Autodesk Inventor part; units mm, degrees
ref_plane "YZ Plane" through (0, 0, 0) normal (1, 0, 0) x (0, 1, 0)
ref_plane "XZ Plane" through (0, 0, 0) normal (0, 1, 0) x (-1, 0, 0)
ref_plane "XY Plane" through (0, 0, 0) normal (0, 0, 1) x (1, 0, 0)
sketch "スケッチ1" plane through (0, 0, 0) normal (0, 0, 1) x (1, 0, 0)
  line L0 (-19.75, 10) -> (19.75, 10) construction
  line L1 (19.75, 10) -> (19.75, -10) construction
  line L2 (19.75, -10) -> (-19.75, -10) construction
  line L3 (-19.75, -10) -> (-19.75, 10) construction
  line L4 (-19.75, 10) -> (19.75, -10) construction
  line L5 (19.75, 10) -> (-19.75, -10) construction
  line L6 (-19.75, 5) -> (-21.75, 5)
  line L7 (-21.75, 5) -> (-21.75, -5)
  line L8 (-19.75, 0) -> (19.75, 0) construction
  line L9 (0, 10) -> (0, -10) construction
  circle A0 centre (0, 0) radius 2.75
  arc A1 (-19.75, 5) -> (-19.75, 7.1) centre (-19.75, 6.05) ccw
  line L10 (-16.75, 10) -> (-11.75, 3)
  line L11 (-19.75, -5) -> (-21.75, -5)
  arc A2 (-19.75, -7.1) -> (-19.75, -5) centre (-19.75, -6.05) ccw
  line L12 (-16.75, -10) -> (-11.75, -3)
  line L13 (-19.75, 7.1) -> (-19.75, 10)
  line L14 (-16.75, 10) -> (-19.75, 10)
  line L15 (-16.75, -10) -> (-19.75, -10)
  line L16 (-19.75, -7.1) -> (-19.75, -10)
  line L17 (19.75, 5) -> (21.75, 5)
  line L18 (21.75, 5) -> (21.75, -5)
  arc A3 (19.75, 7.1) -> (19.75, 5) centre (19.75, 6.05) ccw
  line L19 (16.75, 10) -> (11.75, 3)
  line L20 (19.75, -5) -> (21.75, -5)
  arc A4 (19.75, -5) -> (19.75, -7.1) centre (19.75, -6.05) ccw
  line L21 (16.75, -10) -> (11.75, -3)
  line L22 (19.75, 7.1) -> (19.75, 10)
  line L23 (16.75, 10) -> (19.75, 10)
  line L24 (16.75, -10) -> (19.75, -10)
  line L25 (19.75, -7.1) -> (19.75, -10)
  arc A5 (5.1962, 3) -> (-5.1962, 3) centre (0, 0) ccw
  arc A6 (-5.1962, -3) -> (5.1962, -3) centre (0, 0) ccw
  line L26 (-2.0265, -3.51) -> (-2.5515, -2.6007) construction
  line L27 (-4.053, 0) -> (-3.528, 0.9093) construction
  line L28 (-2.0265, 3.51) -> (-0.9765, 3.51) construction
  line L29 (2.0265, 3.51) -> (2.5515, 2.6007) construction
  line L30 (4.053, 0) -> (3.528, -0.9093) construction
  line L31 (2.0265, -3.51) -> (0.9765, -3.51) construction
  arc A7 (-3.528, 0.9093) -> (-3.528, -0.9093) centre (-3.003, 0) ccw
  arc A8 (-2.5515, -2.6007) -> (-0.9765, -3.51) centre (-1.5015, -2.6007) ccw
  arc A9 (0.9765, -3.51) -> (2.5515, -2.6007) centre (1.5015, -2.6007) ccw
  arc A10 (3.528, -0.9093) -> (3.528, 0.9093) centre (3.003, 0) ccw
  arc A11 (2.5515, 2.6007) -> (0.9765, 3.51) centre (1.5015, 2.6007) ccw
  arc A12 (-0.9765, 3.51) -> (-2.5515, 2.6007) centre (-1.5015, 2.6007) ccw
  line L32 (-2.5515, 2.6007) -> (-2.0265, 3.51) construction
  line L33 (-3.528, 0.9093) -> (-2.5515, 2.6007)
  line L34 (-3.528, -0.9093) -> (-4.053, 0) construction
  line L35 (-2.5515, -2.6007) -> (-3.528, -0.9093)
  line L36 (-0.9765, -3.51) -> (-2.0265, -3.51) construction
  line L37 (0.9765, -3.51) -> (-0.9765, -3.51)
  line L38 (2.5515, -2.6007) -> (2.0265, -3.51) construction
  line L39 (3.528, -0.9093) -> (2.5515, -2.6007)
  line L40 (3.528, 0.9093) -> (4.053, 0) construction
  line L41 (2.5515, 2.6007) -> (3.528, 0.9093)
  line L42 (0.9765, 3.51) -> (2.0265, 3.51) construction
  line L43 (-0.9765, 3.51) -> (0.9765, 3.51)
  line L44 (-11.75, 3) -> (-5.1962, 3)
  line L45 (-5.1962, -3) -> (-11.75, -3)
  line L46 (5.1962, -3) -> (11.75, -3)
  line L47 (11.75, 3) -> (5.1962, 3)
  point P0 (0, 0)
  dimension "d0" = 39.5
  dimension "d3" = 5.5
  dimension "d4" = 2
  dimension "d5" = 10
  dimension "d6" = 1.05
  dimension "d7" = 3
  dimension "d9" = 5
  dimension "d11" = 8
  dimension "d12" = 6
  dimension "d14" = 1.05
  dimension "d17" = 360
  dimension "d19" = 7.02
  dimension "d20" = 6
extrude "押し出し1" add sketch "スケッチ1" along normal blind 3 contours A1 L13 L14 L10 L44 A5 L47 L19 L23 L22 A3 L17 L18 L20 A4 L25 L24 L21 L46 A6 L45 L12 L15 L16 A2 L11 L7 L6
extrude "押し出し2" add sketch "スケッチ1" along normal blind 0.6 contours L33 A12 L43 A11 L41 A10 L39 A9 L37 A8 L35 A7
fillet "フィレット1" radius 2 12 edges at (-11.75, 3, 1.5) (-11.75, -3, 1.5) (-16.75, 10, 1.5) (-16.75, -10, 1.5) (-5.1962, -3, 1.5) (-5.1962, 3, 1.5) (5.1962, 3, 1.5) (5.1962, -3, 1.5) (11.75, 3, 1.5) (11.75, -3, 1.5) (16.75, 10, 1.5) (16.75, -10, 1.5)
properties part number "Ankle_front_frame" material "アルミニウム 2014-T4"
Source: CAD feature listing. Evaluate the final solid. Frame: model axes, mm. A direction names the side the tool comes from. Give positions to 0.01 mm unless a question says otherwise; leave off trailing zeros. Loops run counter-clockwise (first coordinate to the right, second up) from the corner with the lowest first, then second, coordinate; pieces in that order, holes last. Notation, with made-up numbers: (1, 36) -> (16, 36) arc R29 cw to (16, 66) -> close; hole circle Ø6 at (67, -13). An arc over 180 degrees is marked (long way). Use a Markdown table: item, result. Add a question column.
1) Section query B-B, the plane y = -7.5. Return the cut outline in (x, z), then the cut area to 3 significant figures.
2) Reachability of faces 4 (the face through (21, 5, 1)), 5 (the face through (-5.37, -3.2, 1.52)), 6 (the face through (0, 3.51, 2)), 7 (the face through (-21, -5, 1)), 8 (the face through (16.876, 9.784, 1.521)) from +Z, -Z, +X, -X, +Y, -Y: full face, straight path, thin tool, end or side. Return the list, or none.
3) Section query D-D, the plane y = 1.5. Return the cut outline in (x, z).
4) Section query C-C, the plane x = 10. Return the cut outline in (y, z), then the cut area to 3 significant figures.
5) Section query A-A, the plane x = 0. Return the cut outline in (y, z).
6) Line query: line 1 along Y through (x, z) = (19, 2.75); line 2 along X through (y, z) = (-3.75, 2.2); line 3 along X through (y, z) = (-5.5, 2.7). Output: solid intervals per line, ascending. Write a range as [from, to].
7) Pull-direction query (X, two-part tool) for faces 1 (the face through (14.28, 6.54, 1.48)), 2 (the face through (21.75, 0, 1)), 3 (the face through (-5, 0, 3)); classes: +X half, -X half, draft (parallel to the pull), parting line (faces both ways), or undercut.
8) First-contact query: pin 1 (0.9 mm diameter, centred on x = 7.5, z = 1.5, fed in from -Y); pin 2 (7 mm diameter, centred on x = 0, y = 0, fed in from -Z); pin 3 (1.5 mm diameter, centred on y = 8, z = 2, fed in from -X); pin 4 (1 mm diameter, centred on x = 20.5, z = 1, fed in from +Y). Flat tips, straight axial feed; report the tip coordinate or a pass-through.
Numbers:
| question | item | result |
|---|---|---|
| 1 | outline | (-19.75, 0) -> (-14.96, 0) -> (-14.96, 3) -> (-19.75, 3) -> close; (14.96, 0) -> (19.75, 0) -> (19.75, 3) -> (14.96, 3) -> close |
| 1 | area | 28.7 mm2 |
| 2 | face 4 | +Z, -Z, +X, +Y |
| 2 | face 5 | +Z, -Z, -Y |
| 2 | face 6 | +Z |
| 2 | face 7 | +Z, -Z, -X, -Y |
| 2 | face 8 | +Z, -Z, +Y |
| 3 | outline | (-21.75, 0) -> (-2.3, 0) -> (-2.3, 0.6) -> (-3.19, 0.6) -> (-3.19, 3) -> (-21.75, 3) -> close; (2.3, 0) -> (21.75, 0) -> (21.75, 3) -> (3.19, 3) -> (3.19, 0.6) -> (2.3, 0.6) -> close |
| 4 | outline | (-3, 0) -> (3, 0) -> (3, 3) -> (-3, 3) -> close |
| 4 | area | 18.0 mm2 |
| 5 | outline | (-6, 0) -> (-2.75, 0) -> (-2.75, 0.6) -> (-3.51, 0.6) -> (-3.51, 3) -> (-6, 3) -> close; (2.75, 0) -> (6, 0) -> (6, 3) -> (3.51, 3) -> (3.51, 0.6) -> (2.75, 0.6) -> close |
| 6 | line 1 | y = [-10, -6.78], [-5.32, 5.32], [6.78, 10] |
| 6 | line 2 | x = [-21.75, -12.28], [-4.68, 4.68], [12.28, 21.75] |
| 6 | line 3 | x = [-18.86, -13.54], [-2.4, 2.4], [13.54, 18.86] |
| 7 | face 1 | undercut |
| 7 | face 2 | +X half |
| 7 | face 3 | draft |
| 8 | pin 1 | stops at y = -3 |
| 8 | pin 2 | stops at z = 0 |
| 8 | pin 3 | stops at x = -19.75 |
| 8 | pin 4 | stops at y = 5 |
